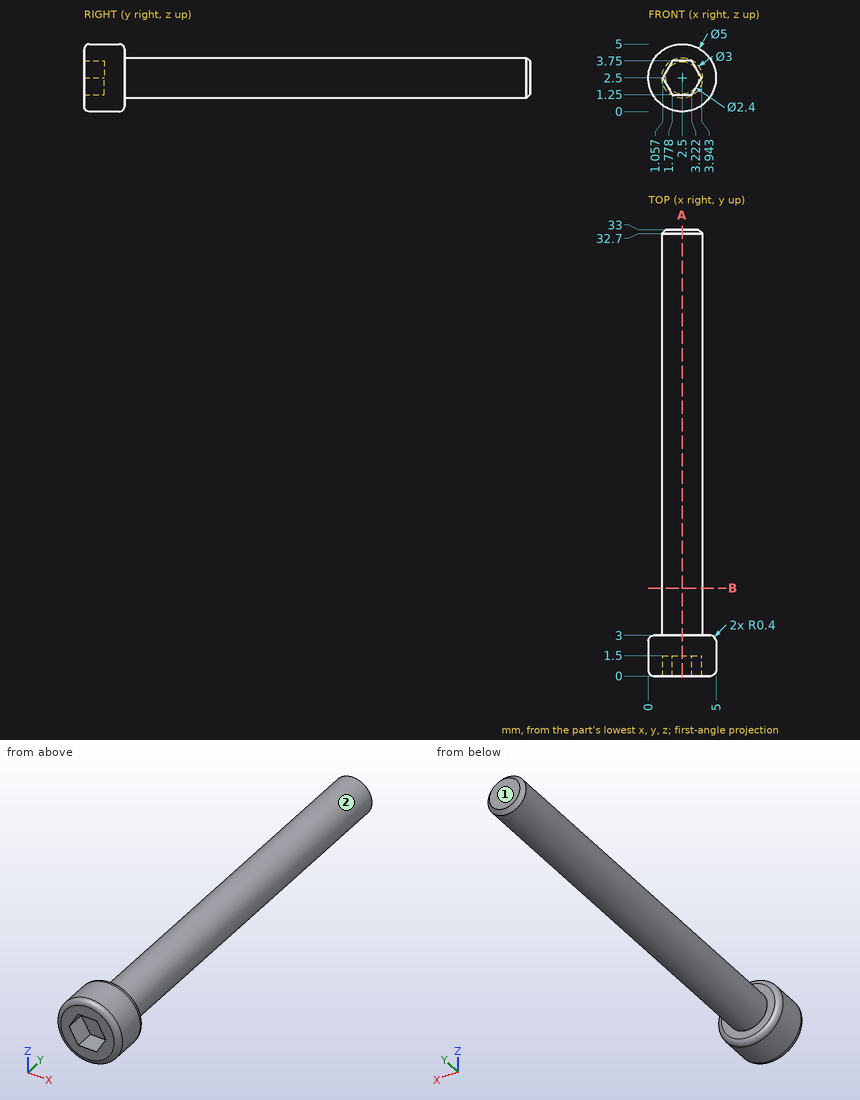
The drawing under review shows one solid part. Ordinate dimensions are in mm from its lowest x, y, z. A direction names the side the tool comes from. Give positions to 0.01 mm unless a question says otherwise; leave off trailing zeros. Loops run counter-clockwise (first coordinate to the right, second up) from the corner with the lowest first, then second, coordinate; pieces in that order, holes last. Notation, with made-up numbers: M 19,-30 L 52,-30 A26 cw 52,1 Z; hole C -6.75,81.5 d4. An arc over 180 degrees is marked long. One line per item, written item: value. Start each with the question number.
Q1. Clearance check with flat-ended pins moving along their axes: pin 1 Ø1 at (x, y) = (4, 6.5) entering from -Z; pin 2 Ø3 at (x, y) = (3, 21.5) entering from +Z; pin 3 Ø3 at (y, z) = (29.5, 4.5) entering from -X (1 decimal). State where each tip first meets the part, or that it passes through.
Q2. Add section A-A (x = 2.5). Give the boundary of the cut face in (y, z).
Q3. For L1, parallel to X at y = 11.5, z = 2.6; L2, parallel to Y at x = 2.25, z = 1.95; L3, parallel to Y at x = 4.05, z = 2.2, list the stretches that pass through material, from the lowest coordinate up.
Q4. Add section B-B (y = 6.5). Give the boundary of the cut face in (x, z).
Q5. Machinability: for the marked faces 1 and 2, which of the approach directions +Z, -Z, +X, -X, +Y, -Y give a long, thin tool a straight path to every point of the face, cutting with its end or side? Answer none if there is none.
Reply:
1. pin 1: z = 1.38
1. pin 2: z = 4
1. pin 3: x = 1.1
2. outline: M 0,0.4 A0.4 ccw 0.4,0 L 2.6,0 A0.4 ccw 3,0.4 L 3,1 L 32.7,1 L 33,1.3 L 33,3.7 L 32.7,4 L 3,4 L 3,4.6 A0.4 ccw 2.6,5 L 0.4,5 A0.4 ccw 0,4.6 L 0,3.75 L 1.5,3.75 L 1.5,1.25 L 0,1.25 Z
3. L1: 1 to 4
3. L2: 1.5 to 33
3. L3: 0 to 3
4. outline: C 2.5,2.5 d3
5. face 1: +Z, -Z, +X, -X, +Y
5. face 2: +Y
